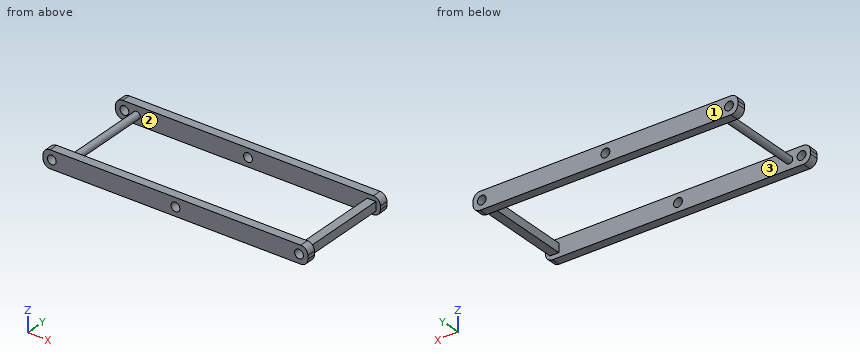
from build123d import *

# Parameters (mm, degrees)
CROQUIS1_W                    = 150
CROQUIS1_H                    = 10
CROQUIS1_R                    = 2.5
SALIENTE_EXTRUIR1_DEPTH       = 5
REDONDEO1_R                   = 4
CROQUIS2_R                    = 2
CROQUIS2_W                    = 5
CROQUIS2_H                    = 5
SALIENTE_EXTRUIR2_DEPTH       = 50
SALIENTE_EXTRUIR2_DEPTH_BACK  = 0.01
CROQUIS3_R                    = 2.5
SALIENTE_EXTRUIR10_DEPTH      = 5
SALIENTE_EXTRUIR10_DEPTH_BACK = 0.001


with BuildPart() as part:
    # Croquis1 → Saliente-Extruir1 (new body)
    with BuildSketch(Plane(origin=(0, 0, 0), x_dir=(1, 0, 0), z_dir=(0, 1, 0))):
        Rectangle(CROQUIS1_W, CROQUIS1_H)
        with Locations((-70, 0)):
            Circle(CROQUIS1_R, mode=Mode.SUBTRACT)
        with Locations((70, 0)):
            Circle(CROQUIS1_R, mode=Mode.SUBTRACT)
        Circle(CROQUIS1_R, mode=Mode.SUBTRACT)
    extrude(amount=SALIENTE_EXTRUIR1_DEPTH)

    # Redondeo1
    redondeo1_edges = [part.edges().sort_by_distance(p)[0] for p in [
        (75, 2.5, 5),
        (-75, 2.5, 5),
        (-75, 2.5, -5),
        (75, 2.5, -5),
    ]]
    fillet(redondeo1_edges, radius=REDONDEO1_R)

    # Croquis2 → Saliente-Extruir2 (add, two sides)
    with BuildSketch(Plane(origin=(0, 5, 0), x_dir=(1, 0, 0), z_dir=(0, 1, 0))) as saliente_extruir2_sk:
        with Locations((-63, 0)):
            Circle(CROQUIS2_R)
        with Locations((70, 0)):
            Rectangle(CROQUIS2_W, CROQUIS2_H)
    extrude(amount=SALIENTE_EXTRUIR2_DEPTH)
    extrude(saliente_extruir2_sk.sketch, amount=-SALIENTE_EXTRUIR2_DEPTH_BACK)

    # Croquis3 → Saliente-Extruir10 (add, two sides)
    with BuildSketch(Plane(origin=(0, 55, 0), x_dir=(1, 0, 0), z_dir=(0, 1, 0))) as saliente_extruir10_sk:
        with BuildLine():
            Line((-75, 1), (-75, -1))
            ThreePointArc((-75, -1), (-73.828427125, -3.828427125), (-71, -5))
            Line((-71, -5), (71, -5))
            ThreePointArc((71, -5), (73.828427125, -3.828427125), (75, -1))
            Line((75, -1), (75, 1))
            ThreePointArc((75, 1), (73.828427125, 3.828427125), (71, 5))
            Line((71, 5), (-71, 5))
            ThreePointArc((-71, 5), (-73.828427125, 3.828427125), (-75, 1))
        make_face()
        with Locations((70, 0)):
            Circle(CROQUIS3_R, mode=Mode.SUBTRACT)
        Circle(CROQUIS3_R, mode=Mode.SUBTRACT)
        with Locations((-70, 0)):
            Circle(CROQUIS3_R, mode=Mode.SUBTRACT)
    extrude(amount=SALIENTE_EXTRUIR10_DEPTH)
    extrude(saliente_extruir10_sk.sketch, amount=-SALIENTE_EXTRUIR10_DEPTH_BACK)


solid = part.part
Geometry: final body of the model. Coordinates: model frame, mm. Face numbers are marked on the shaded views. Coordinates: 2 decimals unless noted, no trailing zeros. Loops run counter-clockwise (first coordinate to the right, second up) from the corner with the lowest first, then second, coordinate; pieces in that order, holes last. Notation, with made-up numbers: (-37, 12.5) - (-10, 12.5) arc R37 cw to (-10, 51.5) - close; hole circle Ø10 at (34.5, 52.5). An arc over 180 degrees is marked (long way). Put each result on its own line as item: value. Start each with the question number.
Q1. Line query: line 1 (X direction, y = 1.35, z = 0); line 2 (Y direction, x = 66.5, z = 4.5); line 3 (Z direction, x = 70, y = 1). Output: solid intervals per line, ascending.
Q2. Cut plane D-D, the plane x = -33. Return loops of the section in (y, z), and give its area (3 significant figures).
Q3. Pull-direction query (X, two-part tool) for the marked faces 1, 2 and 3; classes: released by +X, released by -X, zero draft, split by the parting line, or undercut.
Q4. Cut plane A-A, the plane x = 0. Return loops of the section in (y, z).
Q5. Pin query (flat end, axial travel): pin 1 Ø2.5 at (x, z) = (70.5, -1) entering from +Y; pin 2 Ø1.5 at (x, y) = (71, 24) entering from +Z; pin 3 Ø3 at (x, z) = (-70, 0) entering from +Y; pin 4 Ø6 at (y, z) = (32, -4) entering from +X. Return the tip coordinate at first contact, or that it passes through.
Q6. Cut plane B-B, the plane y = 10. Return loops of the section in (x, z), and give its area (3 significant figures).
Q7. Cut plane C-C, the plane x = -63. Return loops of the section in (y, z), and give its area (3 significant figures).
Filled sheet:
1. line 1: -75 to -72.5, -67.5 to -2.5, 2.5 to 67.5, 72.5 to 75
1. line 2: 0 to 5, 55 to 60
1. line 3: -5 to -2.5, 2.5 to 5
2. outline: (0, -5) - (5, -5) - (5, 5) - (0, 5) - close; (55, -5) - (60, -5) - (60, 5) - (55, 5) - close
2. area: 100 mm²
3. face 1: zero draft
3. face 2: undercut
3. face 3: undercut
4. outline: (0, -5) - (5, -5) - (5, -2.5) - (0, -2.5) - close; (0, 2.5) - (5, 2.5) - (5, 5) - (0, 5) - close; (55, -5) - (60, -5) - (60, -2.5) - (55, -2.5) - close; (55, 2.5) - (60, 2.5) - (60, 5) - (55, 5) - close
5. pin 1: y = 55
5. pin 2: z = 2.5
5. pin 3: through
5. pin 4: x = 72.5
6. outline: circle Ø4 at (-63, 0); (67.5, -2.5) - (72.5, -2.5) - (72.5, 2.5) - (67.5, 2.5) - close
6. area: 37.6 mm²
7. outline: (0, -5) - (5, -5) - (5, -2) - (55, -2) - (55, -5) - (60, -5) - (60, 5) - (55, 5) - (55, 2) - (5, 2) - (5, 5) - (0, 5) - close
7. area: 300 mm²
